Could you check a few things on this model? Use its own coordinates, in mm. A direction names the side the tool comes from. Coordinates: 2 decimals unless noted, no trailing zeros. Write each loop counter-clockwise with the first axis right and the second up, starting at its lowest first coordinate (ties: lowest second). Pieces come first, ordered by that corner, then holes. Notation, with made-up numbers: M 26.25,-8.5 L 77.25,-8.5 A10 cw 77.25,6.5 Z; hole C -17.5,-17 d3. An arc over 180 degrees is marked long. Write item = value, one per line.
```python
from build123d import *

# Parameters (mm, degrees)
ESQUISSE1_R          = 15
BASE_EXTRUSION_DEPTH = 95
CHANFREIN1_SIZE      = 1.5
ESQUISSE2_W          = 55
ESQUISSE2_H          = 5
M_PLAT_DEPTH         = 101.747208398
RAINURE_DEPTH        = 6


with BuildPart() as part:
    # Esquisse1 → Base-Extrusion (new body)
    with BuildSketch(Plane.XY):
        Circle(ESQUISSE1_R)
    extrude(amount=BASE_EXTRUSION_DEPTH)

    # Chanfrein1
    chanfrein1_edges = [part.edges().sort_by_distance(p)[0] for p in [
        (-15, 0, 0),
        (-15, 0, 95),
    ]]
    chamfer(chanfrein1_edges, length=CHANFREIN1_SIZE)

    # Esquisse2 → Méplat (cut, through all)
    with BuildSketch(Plane(origin=(15, 0, 0), x_dir=(0, 0, -1), z_dir=(1, 0, 0))):
        with Locations((-47.5, -15.5)):
            Rectangle(ESQUISSE2_W, ESQUISSE2_H)
    extrude(amount=-M_PLAT_DEPTH, mode=Mode.SUBTRACT)

    # Esquisse3 → Rainure (cut)
    with BuildSketch(Plane.XY.offset(95)):
        Polygon((-10.960155108, -13.788582233), (13.788582233, 10.960155108), (10.960155108, 13.788582233), (-13.788582233, -10.960155108), align=None)
    extrude(amount=-RAINURE_DEPTH, mode=Mode.SUBTRACT)


solid = part.part
```
Item 1: Imagine slicing it at B-B (z = 84). Write out the boundary of the cut face in (x, y), and give its area (3 significant figures).
Numbers:
outline = C 0,0 d30
area = 707 mm²
Item 2: Imagine slicing it at C-C (z = 60.5). Write out the boundary of the cut face in (x, y), and give its area (3 significant figures).
Numbers:
outline = M -7.48,-13 L 7.48,-13 A15 ccw long Z
area = 687 mm²
Item 3: For faces 5 (the face through (-1.953, 14.872, 46.856)), 6 (the face through (0, -14, 20)), 7 (the face through (0, 0, 89)), which set-ups out of +Z, -Z, +X, -X, +Y, -Y let a thin tool reach every point of the face, with its end or its side?
Numbers:
face_5 = +Z, -Z
face_6 = +X, -X, -Y
face_7 = +Z
Item 4: If I drill on line 1 along Y through (x, z) = (0.5, 12.5); line 2 along Z through (x, y) = (-4, -5), over which ranges is the centre line in solid material (lowest first)?
Numbers:
line_1 = -14.99 to 14.99
line_2 = 0 to 89
Item 5: Imagine slicing it at A-A (x = 0). Write out the boundary of the cut face in (y, z), and give its area (3 significant figures).
Numbers:
outline = M -15,1.5 L -13.5,0 L 13.5,0 L 15,1.5 L 15,93.5 L 13.5,95 L 2.83,95 L 2.83,89 L -2.83,89 L -2.83,95 L -13.5,95 L -15,93.5 L -15,75 L -13,75 L -13,20 L -15,20 Z
area = 2,700 mm²
Item 6: If we mould it in two halves opening along Z, with no side actions, what happens to faces 1 (the face through (1.27, -1.56, 92.04)), 2 (the face through (0, -14, 75)), 3 (the face through (9.52, -9.91, 94.76)), 4 (the face through (0, -13, 48))? For each: pulls with the +Z half, pulls with the -Z half, needs draft (parallel to the pull), parting line crosses it, or undercut.
Numbers:
face_1 = needs draft
face_2 = undercut
face_3 = pulls with the +Z half
face_4 = undercut
Item 7: I'm going to push flat-ended pins straight in: P1, Ø1, axis at x = -8.5, z = 51.5, coming from the -Y side; P2, Ø7.5, axis at x = 1, z = 52.5, coming from the -Y side; P3, Ø0.6, axis at x = -3.5, y = -14.5, coming from the +Z side. Where does each tip first touch, or does it pass through?
Numbers:
P1 = -12.69
P2 = -13
P3 = 93.88
